For this review, use the dimensioned drawing (mm, ordinates from the lowest corner) and the shaded views. A direction names the side the tool comes from. Give positions to 0.01 mm unless a question says otherwise; leave off trailing zeros. Write each loop counter-clockwise with the first axis right and the second up, starting at its lowest first coordinate (ties: lowest second). Pieces come first, ordered by that corner, then holes.
1) Machinability: for the marked faces 4, 5, 6 and 7, which of the approach directions +Z, -Z, +X, -X, +Y, -Y give a long, thin tool a straight path to every point of the face, cutting with its end or side? Answer none if there is none.
2) We need section B-B on y = 3.5. Give the boundary of the cut face in (x, z).
3) We need section D-D on z = 7.5. Give the boundary of the cut face in (x, y).
4) Draft analysis for pull direction X (two halves, no side actions). For the marked faces 1, 2 and 3, state which applies: pulls with the +X half, pulls with the -X half, needs draft (parallel to the pull), parting line crosses it, or undercut.
5) Wall thickness on line 1 along X through (y, z) = (15.5, 5.75); line 2 along Z through (x, y) = (8.5, 15); line 3 along Y through (x, z) = (14.25, 6.5): over which ranges is each line inside the solid? List them lowest first.
6) We need section A-A on x = 8.5. Give the boundary of the cut face in (y, z).
7) We need section C-C on z = 17.5. Give the boundary of the cut face in (x, y), and give its area (4 significant figures).
8) For P1, Ø6, axis at x = 10.5, y = 4.5, coming from the +Z side, flat-tipped, find the tip position at first contact; note if it passes through.
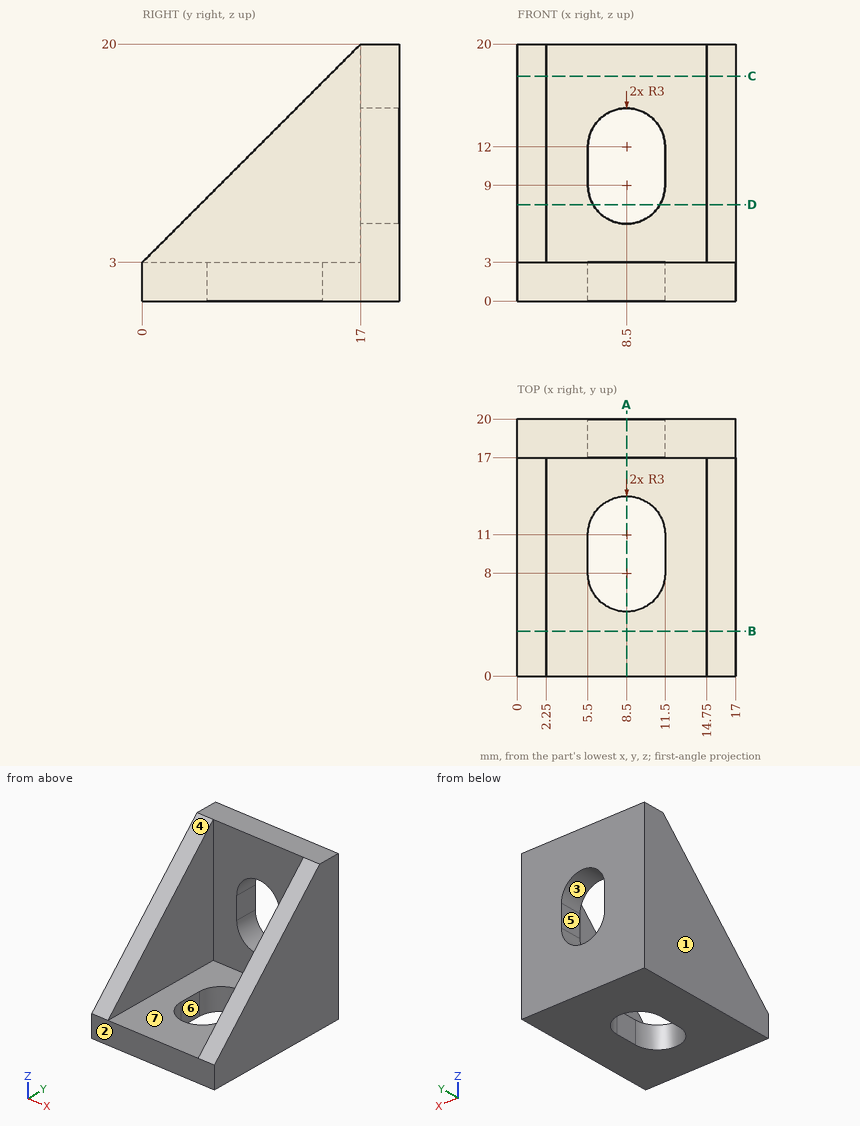
Results list:
1. face 4: +Z, +X, -X, -Y
1. face 5: +Y, -Y
1. face 6: +Z, -Z
1. face 7: +Z, -Y
2. outline: (0, 0) - (17, 0) - (17, 6.5) - (14.75, 6.5) - (14.75, 3) - (2.25, 3) - (2.25, 6.5) - (0, 6.5) - close
3. outline: (0, 4.5) - (2.25, 4.5) - (2.25, 17) - (5.9, 17) - (5.9, 20) - (0, 20) - close; (11.1, 17) - (14.75, 17) - (14.75, 4.5) - (17, 4.5) - (17, 20) - (11.1, 20) - close
4. face 1: pulls with the -X half
4. face 2: needs draft
4. face 3: undercut
5. line 1: x = 0 to 2.25, 14.75 to 17
5. line 2: z = 0 to 3
5. line 3: y = 17 to 20
6. outline: (0, 0) - (5, 0) - (5, 3) - (0, 3) - close; (14, 0) - (20, 0) - (20, 6) - (17, 6) - (17, 3) - (14, 3) - close; (17, 15) - (20, 15) - (20, 20) - (17, 20) - close
7. outline: (0, 14.5) - (2.25, 14.5) - (2.25, 17) - (14.75, 17) - (14.75, 14.5) - (17, 14.5) - (17, 20) - (0, 20) - close
7. area: 62.25 mm2
8. P1: stops at z = 3
